from build123d import *
from OCP.BRepFilletAPI import BRepFilletAPI_MakeChamfer

# Parameters (mm, degrees)
BOSS_EXTRUDE1_DEPTH      = 0.75
BOSS_EXTRUDE1_DEPTH_BACK = 0.75
SKETCH3_R                = 6
SKETCH3_R_2              = 3
CHAMFER1_SIZE            = 0.254
CHAMFER1_SIZE2           = 0.439940905
CHAMFER2_SIZE            = 0.580931391


with BuildPart() as part:
    # Sketch3 → Boss-Extrude1 (new, two sides: drawn at the far end of the back side and taken through both)
    with BuildSketch(Plane.XY.offset(-BOSS_EXTRUDE1_DEPTH_BACK)):
        Circle(SKETCH3_R)
        Circle(SKETCH3_R_2, mode=Mode.SUBTRACT)
    extrude(amount=BOSS_EXTRUDE1_DEPTH + BOSS_EXTRUDE1_DEPTH_BACK)

    # Chamfer1: one chamfer whose edges measure the first distance from different faces: ONE call of the kernel's chamfer builder (chamfer() names one face for all edges)
    chamfer1_edges_1 = [part.edges().sort_by_distance(p)[0] for p in [
        (-6, 0, 0.75),
    ]]
    chamfer1_side_1 = [part.faces().sort_by_distance(p)[0] for p in [
        (-6, 0, 0.375),
    ]]
    chamfer1_edges_2 = [part.edges().sort_by_distance(p)[0] for p in [
        (-6, 0, -0.75),
    ]]
    chamfer1_side_2 = [part.faces().sort_by_distance(p)[0] for p in [
        (-6, 0, -0.375),
    ]]
    chamfer1 = BRepFilletAPI_MakeChamfer(part.part.solid().wrapped)
    for e in chamfer1_edges_1:
        chamfer1.Add(CHAMFER1_SIZE, CHAMFER1_SIZE2, e.wrapped, chamfer1_side_1[0].wrapped)  # the first distance lies on this face
    for e in chamfer1_edges_2:
        chamfer1.Add(CHAMFER1_SIZE, CHAMFER1_SIZE2, e.wrapped, chamfer1_side_2[0].wrapped)  # the first distance lies on this face
    add(Compound.cast(chamfer1.Shape()), mode=Mode.REPLACE)

    # Sketch4 → Cut-Revolve1 (revolve, cut)
    with BuildSketch(Plane(origin=(0, 0, 0), x_dir=(0, 0, -1), z_dir=(1, 0, 0)), mode=Mode.PRIVATE) as cut_revolve1_sk:
        with BuildLine():
            Line((-0.75, 2.9492), (-0.75, 3.0508))
            ThreePointArc((-0.75, 3.0508), (0, 3), (0.75, 3.0508))
            Line((0.75, 3.0508), (0.75, 2.9492))
            Line((0.75, 2.9492), (-0.75, 2.9492))
        make_face()
    revolve(cut_revolve1_sk.sketch.rotate(Axis((0, 0, 0.75), (0, 0, -1)), 90), axis=Axis((0, 0, 0.75), (0, 0, -1)), mode=Mode.SUBTRACT)

    # Chamfer2
    # the kernel refuses this chamfer: 0.580931391, 0.254 mm, written as the material it takes off along each edge
    with BuildSketch(Plane(origin=(0, 0, -0.75), x_dir=(1, 0, 0), z_dir=(0, 1, 0))) as chamfer2_piece_1:
        with BuildLine():
            Line((3.0508 + CHAMFER2_SIZE, 0), (3.022591838, -0.249207666))
            ThreePointArc((3.022591838, -0.249207666), (3.034667103, -0.129981949), (3.0508, 0))
            Line((3.0508, 0), (3.0508 + CHAMFER2_SIZE, 0))
        make_face()
    revolve(axis=Axis((0, 0, -0.75), (0, 0, -1)), mode=Mode.SUBTRACT)
    with BuildSketch(Plane(origin=(0, 0, 0.75), x_dir=(1, 0, 0), z_dir=(0, 1, 0))) as chamfer2_piece_2:
        with BuildLine():
            Line((3.0508 + CHAMFER2_SIZE, 0), (3.022591838, 0.249207666))
            ThreePointArc((3.022591838, 0.249207666), (3.034667103, 0.129981949), (3.0508, 0))
            Line((3.0508, 0), (3.0508 + CHAMFER2_SIZE, 0))
        make_face()
    revolve(axis=Axis((0, 0, 0.75), (0, 0, -1)), mode=Mode.SUBTRACT)


solid = part.part
The model under review builds one solid part; all positions refer to its coordinate system, in mm. Give positions to 0.01 mm unless a question says otherwise; leave off trailing zeros. Loops run counter-clockwise (first coordinate to the right, second up) from the corner with the lowest first, then second, coordinate; pieces in that order, holes last. Notation, with made-up numbers: (-20.75, 56) -> (11.25, 56) arc R34 ccw to (11.25, 93) -> close; hole circle Ø3 at (1.25, 58.25). An arc over 180 degrees is marked (long way). Put each result on its own line as item: value. Start each with the question number.
1. Wall thickness on probe 1 along X at (y, z) = (-1.5, -0.4); probe 2 along Y at (x, z) = (-1.75, 0.2); probe 3 along X at (y, z) = (-2.25, 0.35): over which ranges is each line inside the solid? List them lowest first.
2. We need section A-A on y = 0. State the section outline as (x, z) points, then the cut area to 3 significant figures.
3. We need section C-C on z = 0.25. State the section outline as (x, y) points.
Determined:
1. probe 1: -5.81 to -2.61, 2.61 to 5.81
1. probe 2: -5.74 to -2.44, 2.44 to 5.74
1. probe 3: -5.56 to -2, 2 to 5.56
2. outline: (-6, -0.5) -> (-5.56, -0.75) -> (-3.63, -0.75) -> (-3.02, -0.5) arc R5.56 ccw to (-3.02, 0.5) -> (-3.63, 0.75) -> (-5.56, 0.75) -> (-6, 0.5) -> close; (3.02, -0.5) -> (3.63, -0.75) -> (5.56, -0.75) -> (6, -0.5) -> (6, 0.5) -> (5.56, 0.75) -> (3.63, 0.75) -> (3.02, 0.5) arc R5.56 ccw to start
2. area: 8.44 mm^2
3. outline: circle Ø12 at (0, 0); hole circle Ø6.01 at (0, 0)
